from build123d import *

# Parameters (mm, degrees)
EXTRUDE_1_DEPTH     = 1.5
SKETCH_2_R          = 5
CUT_EXTRUDE_1_DEPTH = 0.5
SKETCH_11_R         = 2
SKETCH_11_W         = 12.230000074
SKETCH_11_H         = 11.97459995
EXTRUDE_5_DEPTH     = 2.539974634
SKETCH_13_R         = 2
SKETCH_13_W         = 4
SKETCH_13_H         = 10
TYPEC_2_DEPTH       = 5.7999746
LED_3_START         = -4.25
LED_3_DEPTH         = 2.75
LED_1_R             = 0.5
CUT_EXTRUDE_2_REACH = 76.258
SKETCH_15_R         = 2
EXTRUDE_START       = -4
SKETCH_16_R         = 4
SKETCH_16_R_2       = 1
SKETCH_16_R_3       = 3.5
SKETCH_16_R_4       = 0.5
EXTRUDE_4_DEPTH     = 2.5
LED_2_START         = -1.5
SKETCH_17_W         = 1
SKETCH_17_H         = 6
LED_2_DEPTH         = 0.5
SKETCH_18_W         = 40.2
SKETCH_18_H         = 3
EXTRUDE_2_DEPTH     = 3.5


with BuildPart() as part:
    # 草图1 → 凸台-拉伸1 (new body)
    with BuildSketch(Plane(origin=(0, 0, 0), x_dir=(1, 0, 0), z_dir=(0, 1, 0))):
        Polygon((-51.714401711, -10.060969859), (-55.976720774, -10.060969859), (-55.976720774, -22.035569809), (-51.714401711, -22.035569809), (-51.714401711, -48.448269834), (46.085598289, -48.448269834), (46.085598289, 16.351730166), (-51.714401711, 16.351730166), align=None)
    extrude(amount=EXTRUDE_1_DEPTH)

    # 草图2 → 防滑切除-拉伸1 (cut)
    with BuildSketch(Plane.XZ):
        with Locations((-43.814401711, 44.448269834)):
            Circle(SKETCH_2_R)
        with Locations((38.185598289, 44.448269834)):
            Circle(SKETCH_2_R)
        with Locations(Location((38.185598289, -8.451730166, 0), (0, 0, 90))):
            Circle(SKETCH_2_R)
        with Locations(Location((-43.814401711, -8.451730166, 0), (0, 0, 270))):
            Circle(SKETCH_2_R)
    extrude(amount=-CUT_EXTRUDE_1_DEPTH, mode=Mode.SUBTRACT)

    # 草图11 → 充电板档板凸台-拉伸5 (add)
    with BuildSketch(Plane.XZ):
        with Locations((-29.074401711, 30.535569809)):
            Circle(SKETCH_11_R)
        with Locations((-29.074401711, 1.560969859)):
            Circle(SKETCH_11_R)
        with Locations((-49.861720737, 16.048269834)):
            Rectangle(SKETCH_11_W, SKETCH_11_H)
    extrude(amount=-EXTRUDE_5_DEPTH)

    # 草图13 → TypeC支撑凸台-拉伸2 (add)
    with BuildSketch(Plane.XZ):
        with Locations(Location((-29.074401711, 30.535569809, 0), (0, 0, 90))):
            Circle(SKETCH_13_R)
        with Locations(Location((-29.074401711, 1.560969859, 0), (0, 0, 90))):
            Circle(SKETCH_13_R)
        with Locations((-46.6267207, 16.048269834)):
            Rectangle(SKETCH_13_W, SKETCH_13_H)
    extrude(amount=-TYPEC_2_DEPTH)

    # 草图14 → LED限位凸台-拉伸3 (add)
    with BuildSketch(Plane.XZ.offset(LED_3_START)):
        Polygon((45.085598289, 13.048269834), (45.085598289, 19.048269834), (46.085598289, 19.048269834), (46.085598289, 22.048269834), (42.085598289, 22.048269834), (42.085598289, 10.048269834), (46.085598289, 10.048269834), (46.085598289, 13.048269834), align=None)
    extrude(amount=LED_3_DEPTH)

    # LED限位圆角1
    led_1_edges = [part.edges().sort_by_distance(p)[0] for p in [
        (-48.6267207, 5.7999746, 16.048269834),
        (45.585598289, 4.25, 19.048269834),
        (45.585598289, 4.25, 13.048269834),
        (45.085598289, 4.25, 16.048269834),
    ]]
    fillet(led_1_edges, radius=LED_1_R)

    # 草图15 → 螺丝孔位切除-拉伸2 (cut, up to next)
    with BuildSketch(Plane.XZ, mode=Mode.PRIVATE) as cut_extrude_2_sk1:
        with Locations(Location((-43.814401711, -8.451730166, 0), (0, 0, 270))):
            Circle(SKETCH_15_R)
    cut_extrude_2_tool1 = extrude(cut_extrude_2_sk1.sketch, amount=-CUT_EXTRUDE_2_REACH, mode=Mode.PRIVATE) & part.part
    # 草图15 → 螺丝孔位切除-拉伸2 (cut, up to next)
    with BuildSketch(Plane.XZ, mode=Mode.PRIVATE) as cut_extrude_2_sk2:
        with Locations(Location((-43.814401711, 44.448269834, 0), (0, 0, 270))):
            Circle(SKETCH_15_R)
    cut_extrude_2_tool2 = extrude(cut_extrude_2_sk2.sketch, amount=-CUT_EXTRUDE_2_REACH, mode=Mode.PRIVATE) & part.part
    # 草图15 → 螺丝孔位切除-拉伸2 (cut, up to next)
    with BuildSketch(Plane.XZ, mode=Mode.PRIVATE) as cut_extrude_2_sk3:
        with Locations(Location((38.185598289, -8.451730166, 0), (0, 0, 270))):
            Circle(SKETCH_15_R)
    cut_extrude_2_tool3 = extrude(cut_extrude_2_sk3.sketch, amount=-CUT_EXTRUDE_2_REACH, mode=Mode.PRIVATE) & part.part
    # 草图15 → 螺丝孔位切除-拉伸2 (cut, up to next)
    with BuildSketch(Plane.XZ, mode=Mode.PRIVATE) as cut_extrude_2_sk4:
        with Locations(Location((38.185598289, 44.448269834, 0), (0, 0, 270))):
            Circle(SKETCH_15_R)
    cut_extrude_2_tool4 = extrude(cut_extrude_2_sk4.sketch, amount=-CUT_EXTRUDE_2_REACH, mode=Mode.PRIVATE) & part.part
    add(cut_extrude_2_tool1.solids().sort_by_distance((-43.814402, 0, -8.45173))[0], mode=Mode.SUBTRACT)
    add(cut_extrude_2_tool2.solids().sort_by_distance((-43.814402, 0, 44.44827))[0], mode=Mode.SUBTRACT)
    add(cut_extrude_2_tool3.solids().sort_by_distance((38.185598, 0, -8.45173))[0], mode=Mode.SUBTRACT)
    add(cut_extrude_2_tool4.solids().sort_by_distance((38.185598, 0, 44.44827))[0], mode=Mode.SUBTRACT)

    # 草图16 → 螺丝孔凸台-拉伸4 (add)
    # profile 1 of 4: a face of its own
    with BuildSketch(Plane.XZ.offset(EXTRUDE_START)):
        with Locations((38.185598289, -8.451730166)):
            Circle(SKETCH_16_R)
        with Locations((38.185598289, -8.451730166)):
            Circle(SKETCH_16_R_2, mode=Mode.SUBTRACT)
    # profile 2 of 4: a face of its own
    with BuildSketch(Plane.XZ.offset(EXTRUDE_START)):
        with Locations((38.185598289, 44.448269834)):
            Circle(SKETCH_16_R)
        with Locations((38.185598289, 44.448269834)):
            Circle(SKETCH_16_R_2, mode=Mode.SUBTRACT)
    # profile 3 of 4: a face of its own
    with BuildSketch(Plane.XZ.offset(EXTRUDE_START)):
        with Locations((-43.814401711, -8.451730166)):
            Circle(SKETCH_16_R)
        with Locations((-43.814401711, -8.451730166)):
            Circle(SKETCH_16_R_2, mode=Mode.SUBTRACT)
    # profile 4 of 4: a face of its own
    with BuildSketch(Plane.XZ.offset(EXTRUDE_START)):
        with Locations((-43.814401711, 44.448269834)):
            Circle(SKETCH_16_R_3)
        with Locations((-43.814401711, 44.448269834)):
            Circle(SKETCH_16_R_4, mode=Mode.SUBTRACT)
    extrude(amount=EXTRUDE_4_DEPTH)

    # 草图17 → LED灯嵌入切除-拉伸2 (cut)
    with BuildSketch(Plane.XZ.offset(LED_2_START)):
        with Locations((45.585598289, 16.048269834)):
            Rectangle(SKETCH_17_W, SKETCH_17_H)
    extrude(amount=LED_2_DEPTH, mode=Mode.SUBTRACT)

    # 草图18 → 散热板支撑凸台-拉伸2 (add)
    with BuildSketch(Plane(origin=(0, 1.5, 0), x_dir=(1, 0, 0), z_dir=(0, 1, 0))):
        with Locations((-5.874401711, 2.451730166)):
            Rectangle(SKETCH_18_W, SKETCH_18_H)
        with Locations((-5.874401711, -34.548269834)):
            Rectangle(SKETCH_18_W, SKETCH_18_H)
    extrude(amount=EXTRUDE_2_DEPTH)


solid = part.part
Part model, mm, in its own coordinate system. A direction names the side the tool comes from. Coordinates: 2 decimals unless noted, no trailing zeros. Loops run counter-clockwise (first coordinate to the right, second up) from the corner with the lowest first, then second, coordinate; pieces in that order, holes last. Notation, with made-up numbers: (7.5, 30.5) -> (20.5, 30.5) arc R20 cw to (20.5, 42.5) -> close; hole circle Ø11 at (78.25, 66). An arc over 180 degrees is marked (long way). Use a Markdown table: item, result. Add a question column.
Item 1: Pull direction X, two halves, no side cores. Call faces 5 (the flat face through (-6, 3, -3.952)), 6 (the cylindrical face through (33.97, 0.25, -5.76)), 7 (the flat face through (46.086, 0.2, 16.2)): +X half, -X half, draft (parallel to the pull), parting line (faces both ways), or undercut.
Item 2: Which spindle directions (+Z, -Z, +X, -X, +Y, -Y) get a long thin tool onto all of the face, cutting with end or side? Do faces 1 (the cylindrical face through (-40, 2.77, -7.25)), 2 (the flat face through (-47, 4, 11.048)), 3 (the flat face through (-6, 3, 33.048)), 4 (the flat face through (44, 4.25, 16)). Say none if no direction does.
Item 3: Band-saw the part on B-B on z = 15.5. Write the cut outline in (x, y).
Item 4: Probe probe 1 along Z at (x, y) = (12, 3.45); probe 2 along X at (y, z) = (1.3, -10); probe 3 along X at (y, z) = (1.95, 45). List the from-to ranges inside material, lowest first.
Item 5: Band-saw the part on C-C on z = 8. Write the cut outline in (x, y), plus the area to 3 significant figures.
Item 6: Flat gauge pins, fed straight in: P1, Ø0.9, axis at y = 2.5, z = 35, coming from the -X side; P2, Ø0.8, axis at y = 2, z = 16.5, coming from the +X side; P3, Ø3.5, axis at x = -52, z = 16.5, coming from the +Y side. Where does each tip first touch, or does it go through?
Item 7: Band-saw the part on A-A on x = -25. Write the cut outline in (y, z), plus the area to 3 significant figures.
Geometry says:
| question | item | result |
|---|---|---|
| 1 | face 5 | draft |
| 1 | face 6 | undercut |
| 1 | face 7 | +X half |
| 2 | face 1 | +Y |
| 2 | face 2 | -X, +Y |
| 2 | face 3 | +X, -X, +Y |
| 2 | face 4 | +Z, -Z, +X, +Y |
| 3 | outline | (-55.98, 0) -> (46.09, 0) -> (46.09, 1) -> (45.09, 1) -> (45.09, 3.75) arc R0.5 ccw to (44.59, 4.25) -> (42.09, 4.25) -> (42.09, 1.5) -> (-43.75, 1.5) -> (-43.75, 2.54) -> (-44.63, 2.54) -> (-44.63, 5.8) -> (-48.13, 5.8) arc R0.5 ccw to (-48.63, 5.3) -> (-48.63, 2.54) -> (-55.98, 2.54) -> close |
| 4 | probe 1 | -3.95 to -0.95, 33.05 to 36.05 |
| 4 | probe 2 | -51.71 to -45.08, -42.55 to 36.92, 39.45 to 46.09 |
| 4 | probe 3 | -47.27 to -40.36, 34.22 to 37.35, 39.02 to 42.15 |
| 5 | outline | (-51.71, 0) -> (46.09, 0) -> (46.09, 1.5) -> (-51.71, 1.5) -> close |
| 5 | area | 147 mm² |
| 6 | P1 | x = -25.97 |
| 6 | P2 | x = 45.09 |
| 6 | P3 | y = 2.54 |
| 7 | outline | (0, -16.35) -> (1.5, -16.35) -> (1.5, -3.95) -> (5, -3.95) -> (5, -0.95) -> (1.5, -0.95) -> (1.5, 33.05) -> (5, 33.05) -> (5, 36.05) -> (1.5, 36.05) -> (1.5, 48.45) -> (0, 48.45) -> close |
| 7 | area | 118 mm² |
